Verification items for this drawing (mm, ordinates from the low corner). Give positions to 0.01 mm unless a question says otherwise; leave off trailing zeros. Order: outer loops, then holes, each group sorted by start corner. A loop starts at its lowest first (then second) coordinate and runs counter-clockwise, first axis right, second up.
(1) Sectioned sample at D-D on y = 6.5. Count the separate pieces of the cut face and the enclosed holes in it, plus the area to 3 significant figures.
(2) Sectioned sample at C-C on x = 27.5. Record the cut outline in (y, z) (1 decimal), plus the area to 3 significant figures.
(3) Sectioned sample at A-A on x = 50.8. Record the cut outline in (y, z), plus the area to 3 significant figures.
(4) Sectioned sample at B-B on z = 44.45. Record the cut outline in (x, y), plus the area to 3 significant figures.
(5) Gauge pin test, flat end, axial feed: pin 1 (20.5 mm diameter, centred on x = 18.16, z = 167.64, fed in from +Y). Record the tip position at first contact, or that the pin passes through.
(6) Scan lines: L1, parallel to Z at x = 50.8, y = 10.25; L2, parallel to Z at x = 19, y = 0.75; L3, parallel to Z at x = 26, y = 9.5. Record each from-to range of solid material in increasing order.
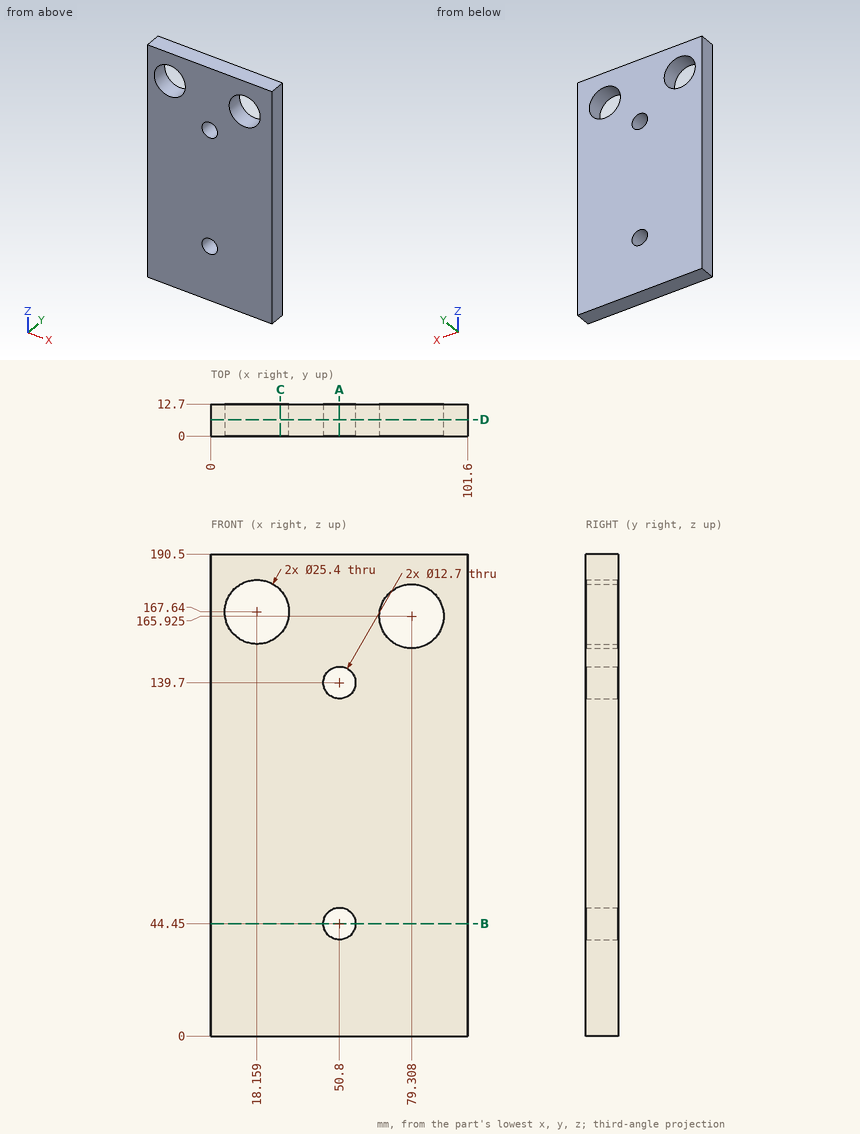
Ans:
1. separate pieces: 1
1. enclosed holes: 4
1. area: 18,100 mm2
2. outline: (0, 0) - (12.7, 0) - (12.7, 159) - (0, 159) - close; (0, 176.2) - (12.7, 176.2) - (12.7, 190.5) - (0, 190.5) - close
2. area: 2,200 mm2
3. outline: (0, 0) - (12.7, 0) - (12.7, 38.1) - (0, 38.1) - close; (0, 50.8) - (12.7, 50.8) - (12.7, 133.35) - (0, 133.35) - close; (0, 146.05) - (12.7, 146.05) - (12.7, 190.5) - (0, 190.5) - close
3. area: 2,100 mm2
4. outline: (0, 0) - (44.45, 0) - (44.45, 12.7) - (0, 12.7) - close; (57.15, 0) - (101.6, 0) - (101.6, 12.7) - (57.15, 12.7) - close
4. area: 1,130 mm2
5. pin 1: passes through
6. L1: z = 0 to 38.1, 50.8 to 133.35, 146.05 to 190.5
6. L2: z = 0 to 154.97, 180.31 to 190.5
6. L3: z = 0 to 157.65, 177.63 to 190.5
